The model under review builds one solid part; all positions refer to its coordinate system, in mm. A direction names the side the tool comes from. Round coordinates to 2 decimals unless told otherwise and drop trailing zeros. Write each loop counter-clockwise with the first axis right and the second up, starting at its lowest first coordinate (ties: lowest second). Pieces come first, ordered by that corner, then holes.
Item 1: Add section A-A (z = -96). Give the boundary of the cut face in (x, y), plus the area to 3 significant figures.
Item 2: Machinability: for faces 5 (the face through (-47.795, 1.479, -12.879)), 6 (the face through (41.56, 1.48, -29.24)), 7 (the face through (-41.7, 1.5, -28.9)), which of the approach directions +Z, -Z, +X, -X, +Y, -Y give a long, thin tool a straight path to every point of the face, cutting with its end or side? Answer none if there is none.
Item 3: Add section D-D (z = -75.5). Give the boundary of the cut face in (x, y).
Item 4: Draft analysis for pull direction Z (two halves, no side actions). For faces 1 (the face through (-33.952, 1.479, -42.934)), 2 (the face through (47.75, 1.48, -13.04)), 3 (the face through (1, 3, -39)), 4 (the face through (0.99, 1.48, 49.49)), state which applies: +Z half, -Z half, draft (parallel to the pull), parting line (faces both ways), or undercut.
Item 5: Add section B-B (x = 18). Give the boundary of the cut face in (y, z).
Item 6: To check wall thickness, follow L1, parallel to X at y = 1.35, z = -42.5; L2, parallel to X at y = 1.1, z = -120; L3, parallel to Z at x = 14, y = 0.7. State the ranges of each line that lie inside material, in increasing order.
Item 7: Add section C-C (y = 1.9). State how many separate pieces and enclosed holes the cut face has, plus the area to 3 significant figures.
Item 8: Clearance check with flat-ended pins moving along their axes: pin 1 Ø1.5 at (x, y) = (-45, 1) entering from +Z; pin 2 Ø0.6 at (x, y) = (38, 1) entering from +Z; pin 3 Ø2.5 at (x, z) = (32, -120) entering from -Y; pin 4 Ø0.6 at (x, y) = (-37.5, 1) entering from +Z. State where each tip first meets the part, or that it passes through.
```python
from build123d import *

# Parameters (mm, degrees)
SKETCH_1_R          = 1.5
SKETCH_1_R_2        = 34
SKETCH_1_R_3        = 2
EXTRUDE_1_DEPTH     = 3
CUT_EXTRUDE_1_DEPTH = 135.477693318
SKETCH_8_R          = 1
CUT_EXTRUDE_3_DEPTH = 135.343775442
FILLET_1_R          = 1
FILLET_2_R          = 5


with BuildPart() as part:
    # 草图1 → Extrude 1 (new body)
    with BuildSketch(Plane(origin=(0, 0, 0), x_dir=(1, 0, 0), z_dir=(0, 1, 0))):
        with BuildLine():
            Line((-37, 40.5), (-37, 52.5))
            Line((-37, 52.5), (-40, 52.5))
            Line((-40, 52.5), (-40, 62.5))
            Line((-40, 62.5), (-37, 62.5))
            Line((-37, 62.5), (-37, 107.5))
            Line((-37, 107.5), (-40, 107.5))
            Line((-40, 107.5), (-40, 117.5))
            Line((-40, 117.5), (-37, 117.5))
            Line((-37, 117.5), (-37, 125))
            Line((-37, 125), (37, 125))
            Line((37, 125), (37, 117.5))
            Line((37, 117.5), (40, 117.5))
            Line((40, 117.5), (40, 107.5))
            Line((40, 107.5), (37, 107.5))
            Line((37, 107.5), (37, 62.5))
            Line((37, 62.5), (40, 62.5))
            Line((40, 62.5), (40, 52.5))
            Line((40, 52.5), (37, 52.5))
            Line((37, 52.5), (37, 40.5))
            Line((37, 40.5), (45.877848892, 18.586903481))
            ThreePointArc((45.877848892, 18.586903481), (0, -49.5), (-45.877848892, 18.586903481))
            Line((-45.877848892, 18.586903481), (-37, 40.5))
        make_face()
        with Locations(Location((-6.35, 45, 0), (0, 0, 270))):
            Circle(SKETCH_1_R, mode=Mode.SUBTRACT)
        with Locations(Location((6.35, 45, 0), (0, 0, 270))):
            Circle(SKETCH_1_R, mode=Mode.SUBTRACT)
        with Locations(Location((0, 85, 0), (0, 0, 270))):
            Circle(SKETCH_1_R_2, mode=Mode.SUBTRACT)
        with Locations(Location((0, 0, 0), (0, 0, 270))):
            Circle(SKETCH_1_R_2, mode=Mode.SUBTRACT)
        with Locations(Location((-32, 120, 0), (0, 0, 270))):
            Circle(SKETCH_1_R, mode=Mode.SUBTRACT)
        with Locations(Location((-32, 42.5, 0), (0, 0, 270))):
            Circle(SKETCH_1_R_3, mode=Mode.SUBTRACT)
        with Locations(Location((32, 42.5, 0), (0, 0, 90))):
            Circle(SKETCH_1_R_3, mode=Mode.SUBTRACT)
        with Locations(Location((32, 120, 0), (0, 0, 90))):
            Circle(SKETCH_1_R, mode=Mode.SUBTRACT)
    extrude(amount=EXTRUDE_1_DEPTH)

    # 草图2 → 切除-拉伸1 (cut, through all)
    with BuildSketch(Plane(origin=(0, 3, 0), x_dir=(1, 0, 0), z_dir=(0, 1, 0))):
        with BuildLine():
            Line((-49.135018062, 6), (-39, 6))
            Line((-39, 6), (-39, -6))
            Line((-39, -6), (-49.135018062, -6))
            ThreePointArc((-49.135018062, -6), (-49.5, 0), (-49.135018062, 6))
        make_face()
        with BuildLine():
            Line((49.135018062, 6), (39, 6))
            Line((39, 6), (39, -6))
            Line((39, -6), (49.135018062, -6))
            ThreePointArc((49.135018062, -6), (49.5, 0), (49.135018062, 6))
        make_face()
    extrude(amount=-CUT_EXTRUDE_1_DEPTH, mode=Mode.SUBTRACT)

    # 草图8 → 切除-拉伸3 (cut, through all)
    with BuildSketch(Plane(origin=(0, 3, 0), x_dir=(1, 0, 0), z_dir=(0, 1, 0))):
        with Locations((-37, 118.5)):
            Circle(SKETCH_8_R)
        with Locations((-37, 106.5)):
            Circle(SKETCH_8_R)
        with Locations((-37, 63.5)):
            Circle(SKETCH_8_R)
        with Locations((-37, 51.5)):
            Circle(SKETCH_8_R)
        with Locations((37, 51.5)):
            Circle(SKETCH_8_R)
        with Locations((37, 63.5)):
            Circle(SKETCH_8_R)
        with Locations((37, 106.5)):
            Circle(SKETCH_8_R)
        with Locations((37, 118.5)):
            Circle(SKETCH_8_R)
    extrude(amount=-CUT_EXTRUDE_3_DEPTH, mode=Mode.SUBTRACT)

    # 圆角1
    fillet_1_edges = [part.edges().sort_by_distance(p)[0] for p in [
        (-49.135018062, 1.5, 6),
        (-49.135018062, 1.5, -6),
        (-39, 1.5, -6),
        (-39, 1.5, 6),
        (49.135018062, 1.5, -6),
        (49.135018062, 1.5, 6),
        (39, 1.5, 6),
        (39, 1.5, -6),
        (-40, 1.5, -107.5),
        (-40, 1.5, -117.5),
        (-37, 1.5, -125),
        (37, 1.5, -125),
        (40, 1.5, -117.5),
        (40, 1.5, -107.5),
        (40, 1.5, -62.5),
        (40, 1.5, -52.5),
        (-40, 1.5, -52.5),
        (-40, 1.5, -62.5),
    ]]
    fillet(fillet_1_edges, radius=FILLET_1_R)

    # 圆角2
    fillet_2_edges = [part.edges().sort_by_distance(p)[0] for p in [
        (37, 1.5, -40.5),
        (-37, 1.5, -40.5),
    ]]
    fillet(fillet_2_edges, radius=FILLET_2_R)


solid = part.part
```
Numbers:
1. outline: (-37, 0) - (-32.17, 0) - (-32.17, 3) - (-37, 3) - close; (32.17, 0) - (37, 0) - (37, 3) - (32.17, 3) - close
1. area: 29.0 mm2
2. face 5: -Z, -X, +Y, -Y
2. face 6: +X, +Y, -Y
2. face 7: -X, +Y, -Y
3. outline: (-37, 0) - (-32.65, 0) - (-32.65, 3) - (-37, 3) - close; (32.65, 0) - (37, 0) - (37, 3) - (32.65, 3) - close
4. face 1: undercut
4. face 2: -Z half
4. face 3: draft
4. face 4: +Z half
5. outline: (0, -125) - (3, -125) - (3, -113.84) - (0, -113.84) - close; (0, -56.16) - (3, -56.16) - (3, -28.84) - (0, -28.84) - close; (0, 28.84) - (3, 28.84) - (3, 46.11) - (0, 46.11) - close
6. L1: x = -37 to -34, -30 to 30, 34 to 37
6. L2: x = -37 to -33.5, -30.5 to 30.5, 33.5 to 37
6. L3: z = -125 to -115.98, -54.02 to -30.98, 30.98 to 47.48
7. separate pieces: 1
7. enclosed holes: 8
7. area: 6,250 mm2
8. pin 1: stops at z = 22.19
8. pin 2: stops at z = 32.08
8. pin 3: passes through
8. pin 4: stops at z = 32.66
